Read the model definition and answer for the solid it produces. Units are mm, in the model's axes. A direction names the side the tool comes from. Round coordinates to 2 decimals unless told otherwise and drop trailing zeros. Write each loop counter-clockwise with the first axis right and the second up, starting at its lowest first coordinate (ties: lowest second). Pieces come first, ordered by that corner, then holes. Notation, with made-up numbers: (-32.75, 59) - (-28.75, 59) arc R24 ccw to (-28.75, 73) - close; hole circle Ø5 at (64, -38.75). An arc over 180 degrees is marked (long way). Use one line per item in the form item = value. Start each with the question number.
1) For a pull along Z with two mould halves and no side action, classify faces 1 (the face through (76.2, 2, -6)), 2 (the face through (38, 2, 0)), 3 (the face through (0, 2, -32)) as released by +Z, released by -Z, zero draft, split by the parting line, or undercut.
2) Each of these flat-tipped pins is pushed along its axis until it touches: pin 1 (1 mm diameter, centred on y = 2.5, z = -2.5, fed in from +X); pin 2 (1 mm diameter, centred on x = 78.5, y = 2, fed in from +Z); pin 3 (1.6 mm diameter, centred on y = 1, z = -85, fed in from -X). Where does it stop, or does it pass through?
3) For faces 4 (the face through (78, 2, -38.1)), 5 (the face through (0, 2, -6)), 6 (the face through (47.625, 2, -2)), 7 (the face through (-2, 2, -50.8)), determine the directions among +Z, -Z, +X, -X, +Y, -Y from which every point of the face is accessible in a straight line to the end or side of a thin tool.
4) The part is cut by section A-A, the plane x = 46. Give the vertices of the cut face in (y, z) (3 decimals).
5) Consider line 1 along X through (y, z) = (0.75, -88.5); line 2 along Z through (x, y) = (42.5, 0.7) (3 decimals). Determine where each line is inside the solid, lowest interval first. Write a range as from..to.
6) The part is cut by section B-B, the plane z = -7.5. Give the vertices of the cut face in (x, y) (3 decimals), plus the area to 3 significant figures.
from build123d import *

# Parameters (mm, degrees)
BOSS_EXTRUDE1_DEPTH = 3.175
SKETCH2_W           = 6.35
SKETCH2_H           = 3.175
CUT_EXTRUDE1_DEPTH  = 4.175


with BuildPart() as part:
    # Sketch1 → Boss-Extrude1 (new body)
    with BuildSketch(Plane(origin=(0, 0, 0), x_dir=(1, 0, 0), z_dir=(0, 1, 0))):
        Polygon((0, 0), (76.2, 0), (76.2, 12.7), (79.375, 12.7), (79.375, 25.4), (76.2, 25.4), (76.2, 38.1), (79.375, 38.1), (79.375, 50.8), (76.2, 50.8), (76.2, 63.5), (79.375, 63.5), (79.375, 76.2), (76.2, 76.2), (76.2, 88.9), (79.375, 88.9), (79.375, 101.6), (-3.175, 101.6), (-3.175, 88.9), (0, 88.9), (0, 76.2), (-3.175, 76.2), (-3.175, 63.5), (0, 63.5), (0, 50.8), (-3.175, 50.8), (-3.175, 38.1), (0, 38.1), (0, 25.4), (-3.175, 25.4), (-3.175, 12.7), (0, 12.7), align=None)
    extrude(amount=BOSS_EXTRUDE1_DEPTH)

    # Sketch2 → Cut-Extrude1 (cut, through all)
    with BuildSketch(Plane(origin=(0, 3.175, 0), x_dir=(1, 0, 0), z_dir=(0, 1, 0))):
        with Locations((44.45, 1.5875)):
            Rectangle(SKETCH2_W, SKETCH2_H)
        with Locations((31.75, 1.5875)):
            Rectangle(SKETCH2_W, SKETCH2_H)
    extrude(amount=-CUT_EXTRUDE1_DEPTH, mode=Mode.SUBTRACT)


solid = part.part
Geometry results:
q1.face_1 = zero draft
q1.face_2 = released by +Z
q1.face_3 = undercut
q2.pin_1 = 76.2
q2.pin_2 = -12.7
q2.pin_3 = 0
q3.face_4 = +X, +Y, -Y
q3.face_5 = +Z, -X, +Y, -Y
q3.face_6 = +Z, +Y, -Y
q3.face_7 = -X, +Y, -Y
q4.outline = (0, -101.6) - (3.175, -101.6) - (3.175, -3.175) - (0, -3.175) - close
q5.line_1 = 0..76.2
q5.line_2 = -101.6..-3.175
q6.outline = (0, 0) - (76.2, 0) - (76.2, 3.175) - (0, 3.175) - close
q6.area = 242 mm2
